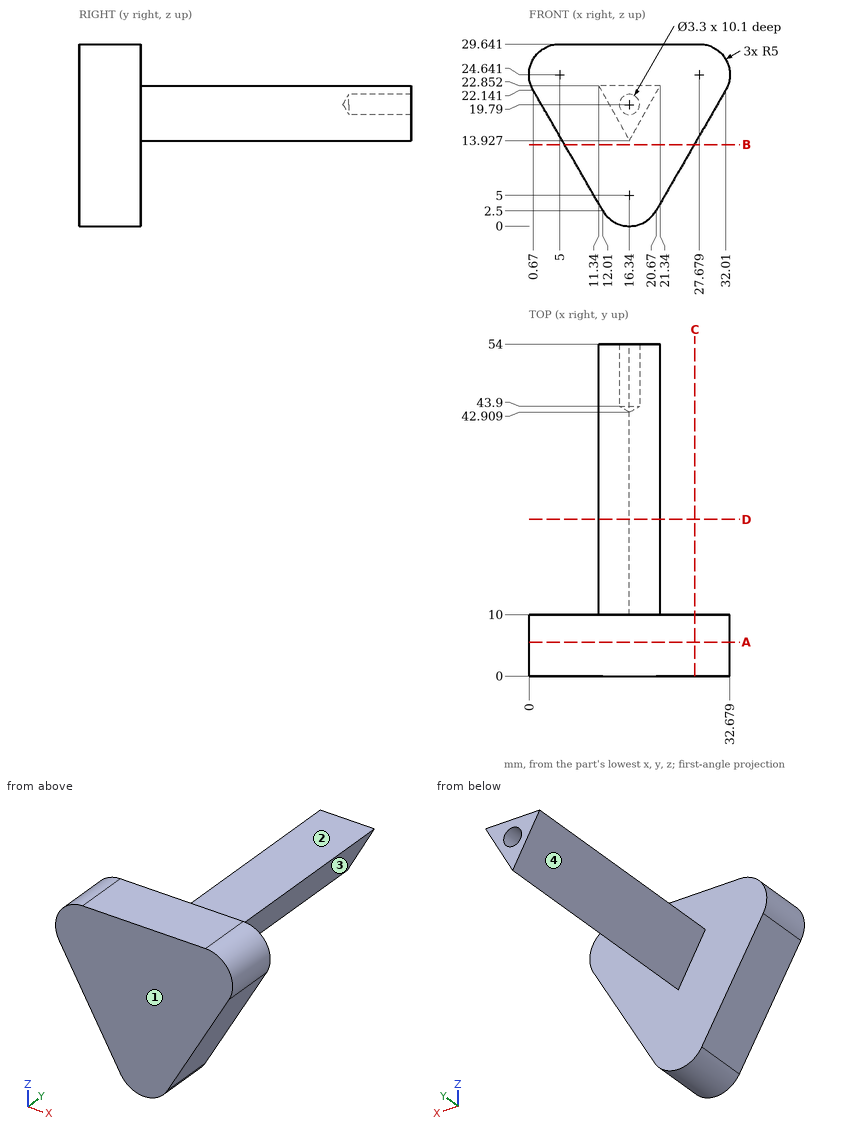
Can you work these out from the drawing? Everything is in mm from the part's minimum corner. A direction names the side the tool comes from. Give positions to 0.01 mm unless a question says otherwise; leave off trailing zeros. Order: outer loops, then holes, each group sorted by start corner. A loop starts at its lowest first (then second) coordinate and runs counter-clockwise, first axis right, second up.
Item 1: I need wall thicknesses on line 1 (Y direction, x = 29.5, z = 20.25); line 2 (X direction, y = 26, z = 18.5); line 3 (X direction, y = 34.5, z = 22) (1 decimal). Which ranges of each line are inside material? Lowest first, please.
Item 2: If we section it at B-B, the plane z = 13.25: Write out the boundary of the cut face in (x, y).
Item 3: I'm going to push flat-ended pins straight in: pin 1 (3 mm diameter, centred on x = 10.5, z = 22, fed in from -Y); pin 2 (6 mm diameter, centred on y = 15.5, z = 21.5, fed in from -X); pin 3 (1.5 mm diameter, centred on x = 10, z = 16, fed in from +Y); pin 4 (5 mm diameter, centred on x = 15, y = 35.5, fed in from +Z). Where does each tip first touch, or does it pass through?
Item 4: If we section it at A-A, the plane y = 5.5: Write out the boundary of the cut face in (x, z).
Item 5: If we section it at C-C, the plane x = 27: Write out the boundary of the cut face in (y, z) (1 decimal), plus the area to 3 significant figures.
Item 6: If we section it at D-D, the plane y = 25.5: Write out the boundary of the cut face in (x, z).
Item 7: For the marked faces 1, 2, 3 and 4, which set-ups out of +Z, -Z, +X, -X, +Y, -Y let a thin tool reach every point of the face, with its end or its side?
Values:
1. line 1: y = 0 to 10
1. line 2: x = 13.78 to 18.9
1. line 3: x = 11.8 to 20.9
2. outline: (5.8, 0) - (26.88, 0) - (26.88, 10) - (5.8, 10) - close
3. pin 1: stops at y = 0
3. pin 2: stops at x = 11.34
3. pin 3: stops at y = 10
3. pin 4: stops at z = 22.85
4. outline: (0.67, 22.14) - (12.01, 2.5) arc R5 ccw to (20.67, 2.5) - (32.01, 22.14) arc R5 ccw to (27.68, 29.64) - (5, 29.64) arc R5 ccw to start
5. outline: (0, 13.5) - (10, 13.5) - (10, 29.6) - (0, 29.6) - close
5. area: 162 mm2
6. outline: (11.34, 22.85) - (16.34, 13.93) - (21.34, 22.85) - close
7. face 1: +Z, -Z, +X, -X, -Y
7. face 2: +Z, +X, -X, +Y
7. face 3: -Z, +X, +Y
7. face 4: -Z, -X, +Y
